Geometry check sheet. Reference: the model listing, model coordinates, mm. A direction names the side the tool comes from. Give positions to 0.01 mm unless a question says otherwise; leave off trailing zeros. Loops run counter-clockwise (first coordinate to the right, second up) from the corner with the lowest first, then second, coordinate; pieces in that order, holes last. Notation, with made-up numbers: (59, 81.25) -> (100, 81.25) arc R33 cw to (100, 120.25) -> close; hole circle Ø1 at (82, 60). An arc over 180 degrees is marked (long way). Answer in a Markdown table with one row per item. Add a question column.
```python
from build123d import *

# Parameters (mm, degrees)
SKETCH1_W           = 145
SKETCH1_H           = 18
BOSS_EXTRUDE1_DEPTH = 3.8
SKETCH2_W           = 10
SKETCH2_H           = 3.8
SKETCH2_H_2         = 7.6
BOSS_EXTRUDE2_DEPTH = 3.8
LPATTERN1_COUNT     = 4
LPATTERN1_PITCH     = 20
LPATTERN1_COL_COUNT = 4
LPATTERN1_COL_PITCH = 20
SKETCH3_W           = 145
SKETCH3_H           = 3
BOSS_EXTRUDE3_DEPTH = 3.8
SKETCH4_W           = 10
SKETCH4_H           = 3.8
CUT_EXTRUDE1_DEPTH  = 148.154612568
SKETCH5_W           = 12.8
SKETCH5_H           = 3
CUT_EXTRUDE2_DEPTH  = 148.154612568
SKETCH6_W           = 3.8
SKETCH6_H           = 8
CUT_EXTRUDE3_DEPTH  = 148.154612568


with BuildPart() as part:
    # Sketch1 → Boss-Extrude1 (new body)
    with BuildSketch(Plane(origin=(0, 0, 0), x_dir=(1, 0, 0), z_dir=(0, 1, 0))):
        with Locations((72.5, -9)):
            Rectangle(SKETCH1_W, SKETCH1_H)
    extrude(amount=BOSS_EXTRUDE1_DEPTH)

    # Sketch2 → Boss-Extrude2 (add, through all)
    with BuildSketch(Plane.XZ):
        with Locations((72.5, 19.9)):
            Rectangle(SKETCH2_W, SKETCH2_H)
        with Locations((72.5, -3.8)):
            Rectangle(SKETCH2_W, SKETCH2_H_2)
    boss_extrude2 = extrude(amount=-BOSS_EXTRUDE2_DEPTH)

    # LPattern1: Boss-Extrude2 ×4
    with Locations(*[(i * LPATTERN1_PITCH, 0, 0) for i in range(1, LPATTERN1_COUNT)]):
        add(boss_extrude2)

    # LPattern1 col: Boss-Extrude2 ×4
    with Locations(*[(-i * LPATTERN1_COL_PITCH, 0, 0) for i in range(1, LPATTERN1_COL_COUNT)]):
        add(boss_extrude2)

    # Sketch3 → Boss-Extrude3 (add, through all)
    with BuildSketch(Plane(origin=(0, 3.8, 0), x_dir=(1, 0, 0), z_dir=(0, 1, 0))):
        with Locations((72.5, -23.3)):
            Rectangle(SKETCH3_W, SKETCH3_H)
    extrude(amount=-BOSS_EXTRUDE3_DEPTH)

    # Sketch4 → Cut-Extrude1 (cut, through all)
    with BuildSketch(Plane(origin=(0, 3.8, 0), x_dir=(1, 0, 0), z_dir=(0, 1, 0))):
        with Locations((12.5, -19.9)):
            Rectangle(SKETCH4_W, SKETCH4_H)
        with Locations((132.5, -19.9)):
            Rectangle(SKETCH4_W, SKETCH4_H)
    extrude(amount=-CUT_EXTRUDE1_DEPTH, mode=Mode.SUBTRACT)

    # Sketch5 → Cut-Extrude2 (cut, through all)
    with BuildSketch(Plane(origin=(0, 3.8, 0), x_dir=(1, 0, 0), z_dir=(0, 1, 0))):
        with Locations((6.4, -23.3)):
            Rectangle(SKETCH5_W, SKETCH5_H)
        with Locations((138.6, -23.3)):
            Rectangle(SKETCH5_W, SKETCH5_H)
    extrude(amount=-CUT_EXTRUDE2_DEPTH, mode=Mode.SUBTRACT)

    # Sketch6 → Cut-Extrude3 (cut, through all)
    with BuildSketch(Plane.XZ):
        with Locations((1.9, 9)):
            Rectangle(SKETCH6_W, SKETCH6_H)
        with Locations((143.1, 9)):
            Rectangle(SKETCH6_W, SKETCH6_H)
    extrude(amount=-CUT_EXTRUDE3_DEPTH, mode=Mode.SUBTRACT)


solid = part.part
```
1. Material ranges on L1, parallel to X at y = 1.65, z = 20; L2, parallel to Z at x = 84.5, y = 1.65; L3, parallel to Z at x = 131, y = 2.4, recorded low to high. Write a range as from..to.
2. Sectioned sample at C-C (x = 16). Enter the section's corners in (y, z), plus the area to 3 significant figures.
3. Gauge pin test, flat ends, axial feed: pin 1 Ø1.9 at (x, y) = (143, 1) entering from -Z; pin 2 Ø1.1 at (y, z) = (2, -3.5) entering from -X; pin 3 Ø1.1 at (y, z) = (2.5, 21) entering from +X. Record the tip position at first contact, or that the pin passes through.
4. Sectioned sample at B-B (x = 125). Enter the section's corners in (y, z), plus the area to 3 significant figures.
5. Access from +Z, -Z, +X, -X, +Y, -Y to the whole of each face (thin tool, end or side, straight path). Record for faces 4 (the face through (107.5, 2, 20)), 5 (the face through (143, 2, 5)), 6 (the face through (7.5, 2, -4)), 7 (the face through (17.5, 2, -4)).
6. Release check for a two-part mould opening along X. For faces 1 (the face through (27.5, 2, 20)), 2 (the face through (37.5, 2, 20)), 3 (the face through (141.2, 2, 9)) record: released by +X, released by -X, zero draft, split by the parting line, or undercut.
7. Sectioned sample at A-A (z = -3). Enter the section's corners in (x, y), plus the area to 3 significant figures.
8. Sectioned sample at D-D (y = 2). Count the separate pieces of the cut face and the enclosed holes in it, plus the area to 3 significant figures.
Response:
| question | item | result |
|---|---|---|
| 1 | L1 | x = 27.5..37.5, 47.5..57.5, 67.5..77.5, 87.5..97.5, 107.5..117.5 |
| 1 | L2 | z = 0..18, 21.8..24.8 |
| 1 | L3 | z = -7.6..18, 21.8..24.8 |
| 2 | outline | (0, -7.6) -> (3.8, -7.6) -> (3.8, 18) -> (0, 18) -> close; (0, 21.8) -> (3.8, 21.8) -> (3.8, 24.8) -> (0, 24.8) -> close |
| 2 | area | 109 mm2 |
| 3 | pin 1 | stops at z = 0 |
| 3 | pin 2 | stops at x = 7.5 |
| 3 | pin 3 | stops at x = 117.5 |
| 4 | outline | (0, 0) -> (3.8, 0) -> (3.8, 18) -> (0, 18) -> close; (0, 21.8) -> (3.8, 21.8) -> (3.8, 24.8) -> (0, 24.8) -> close |
| 4 | area | 79.8 mm2 |
| 5 | face 4 | +Y, -Y |
| 5 | face 5 | +X, +Y, -Y |
| 5 | face 6 | -Z, -X, +Y, -Y |
| 5 | face 7 | -Z, +Y, -Y |
| 6 | face 1 | released by -X |
| 6 | face 2 | undercut |
| 6 | face 3 | released by +X |
| 7 | outline | (7.5, 0) -> (17.5, 0) -> (17.5, 3.8) -> (7.5, 3.8) -> close; (27.5, 0) -> (37.5, 0) -> (37.5, 3.8) -> (27.5, 3.8) -> close; (47.5, 0) -> (57.5, 0) -> (57.5, 3.8) -> (47.5, 3.8) -> close; (67.5, 0) -> (77.5, 0) -> (77.5, 3.8) -> (67.5, 3.8) -> close; (87.5, 0) -> (97.5, 0) -> (97.5, 3.8) -> (87.5, 3.8) -> close; (107.5, 0) -> (117.5, 0) -> (117.5, 3.8) -> (107.5, 3.8) -> close; (127.5, 0) -> (137.5, 0) -> (137.5, 3.8) -> (127.5, 3.8) -> close |
| 7 | area | 266 mm2 |
| 8 | separate pieces | 1 |
| 8 | enclosed holes | 4 |
| 8 | area | 3,630 mm2 |
